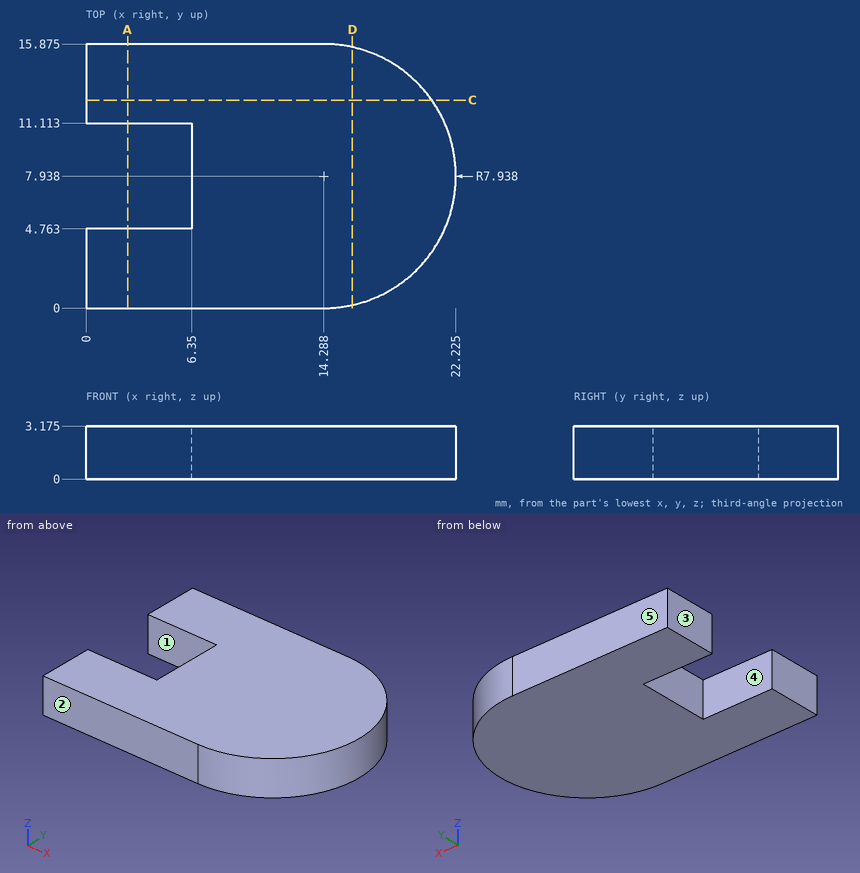
Check sheet for the drawn part. Datum: minimum x, y, z corner. Units: mm. A direction names the side the tool comes from. Give positions to 0.01 mm unless a question says otherwise; leave off trailing zeros. Order: outer loops, then holes, each group sorted by start corner. A loop starts at its lowest first (then second) coordinate and runs counter-clockwise, first axis right, second up. Notation, with made-up numbers: (3.5, 41) - (11.5, 41) arc R22 ccw to (11.5, 52) - close; hole circle Ø1 at (4, -0.5). An arc over 180 degrees is marked (long way). Write item = value, one per line. Start each with the question number.
1) Section check D-D (x = 16). Enter the section's corners in (y, z) (1 decimal).
2) Section check C-C (y = 12.5). Enter the section's corners in (x, z) (1 decimal).
3) Draft check along Y on the marked faces 3, 4 and 5. Enter one of: released by +Y, released by -Y, zero draft, split by the parting line, or undercut.
4) Access from +Z, -Z, +X, -X, +Y, -Y to the whole of each face (thin tool, end or side, straight path). Record for the marked faces 1 and 2.
5) Scan lines: L1, parallel to Y at x = 4.25, z = 1.1 (1 decimal); L2, parallel to Y at x = 14.5, z = 2.95; L3, parallel to X at y = 10.75, z = 0.5. Record each from-to range of solid material in increasing order.
6) Section check A-A (x = 2.5). Enter the section's corners in (y, z) (1 decimal).
Geometry check:
q1.outline = (0.2, 0) - (15.7, 0) - (15.7, 3.2) - (0.2, 3.2) - close
q2.outline = (0, 0) - (20.8, 0) - (20.8, 3.2) - (0, 3.2) - close
q3.face_3 = zero draft
q3.face_4 = undercut
q3.face_5 = released by +Y
q4.face_1 = +Z, -Z, -X
q4.face_2 = +Z, -Z, +X, -X, -Y
q5.L1 = 0 to 4.8, 11.1 to 15.9
q5.L2 = 0 to 15.87
q5.L3 = 6.35 to 21.71
q6.outline = (0, 0) - (4.8, 0) - (4.8, 3.2) - (0, 3.2) - close; (11.1, 0) - (15.9, 0) - (15.9, 3.2) - (11.1, 3.2) - close
